```python
from build123d import *

# Parameters (mm, degrees)
BOSS_EXTRUDE1_DEPTH      = 8.83
BOSS_EXTRUDE1_DEPTH_BACK = 3.83
SKETCH1_W                = 35.75
SKETCH1_H                = 30
SKETCH1_R                = 1.725
SKETCH2_W                = 31.75
SKETCH2_H                = 4.83
CUT_EXTRUDE1_DEPTH       = 37.317668183
BOSS_EXTRUDE4_DEPTH      = 7.368601
BOSS_EXTRUDE4_DEPTH_BACK = 22.631399
SKETCH7_W                = 25.4
SKETCH7_H                = 1.05
CUT_EXTRUDE2_DEPTH       = 73.49839785
SKETCH8_R                = 2.85
CUT_EXTRUDE3_DEPTH       = 3


with BuildPart() as part:
    # Sketch1 → Boss-Extrude1 (new, two sides: drawn at the far end of the back side and taken through both)
    with BuildSketch(Plane(origin=(0, 0, 0), x_dir=(1, 0, 0), z_dir=(0, 1, 0)).offset(-BOSS_EXTRUDE1_DEPTH_BACK)):
        with Locations((-0.591296928, 7.631399317)):
            Rectangle(SKETCH1_W, SKETCH1_H)
        with Locations(Location((-0.591296928, 7.631399317, 0), (0, 0, 270))):
            Circle(SKETCH1_R, mode=Mode.SUBTRACT)
    extrude(amount=BOSS_EXTRUDE1_DEPTH + BOSS_EXTRUDE1_DEPTH_BACK)

    # Sketch2 → Cut-Extrude1 (cut, through all)
    with BuildSketch(Plane(origin=(0, 0, -22.631399317), x_dir=(-1, 0, 0), z_dir=(0, 0, -1))):
        with Locations((0.591296928, 2.5)):
            Rectangle(SKETCH2_W, SKETCH2_H)
    extrude(amount=-CUT_EXTRUDE1_DEPTH, mode=Mode.SUBTRACT)

    # Sketch4 → Boss-Extrude4 (add, two sides: drawn at the far end of the back side and taken through both)
    with BuildSketch(Plane.XY.offset(-BOSS_EXTRUDE4_DEPTH_BACK)):
        with BuildLine():
            Line((33.562284713, -6.212446851), (19.98770661, -6.212446851))
            ThreePointArc((19.98770661, -6.212446851), (18.67257107, -4.979381394), (17.283703072, -3.83))
            Line((17.283703072, -3.83), (17.283703072, 8.83))
            ThreePointArc((17.283703072, 8.83), (26.488439568, 2.461776787), (33.562284713, -6.212446851))
        make_face()
        with BuildLine():
            Line((-21.170300466, -6.212446851), (-34.74487857, -6.212446851))
            ThreePointArc((-34.74487857, -6.212446851), (-27.671033425, 2.461776787), (-18.466296928, 8.83))
            Line((-18.466296928, 8.83), (-18.466296928, -3.83))
            ThreePointArc((-18.466296928, -3.83), (-19.855164927, -4.979381394), (-21.170300466, -6.212446851))
        make_face()
    extrude(amount=BOSS_EXTRUDE4_DEPTH + BOSS_EXTRUDE4_DEPTH_BACK)

    # Sketch7 → Cut-Extrude2 (cut, through all)
    with BuildSketch(Plane.ZY.offset(34.74487857)):
        with Locations((-7.631399317, -4.340632565)):
            Rectangle(SKETCH7_W, SKETCH7_H)
    extrude(amount=-CUT_EXTRUDE2_DEPTH, mode=Mode.SUBTRACT)

    # Sketch8 → Cut-Extrude3 (cut)
    with BuildSketch(Plane.XZ.offset(3.83)):
        with Locations(Location((-0.591296928, -7.631399317, 0), (0, 0, 270))):
            Circle(SKETCH8_R)
    extrude(amount=-CUT_EXTRUDE3_DEPTH, mode=Mode.SUBTRACT)


solid = part.part
```
The model under review builds one solid part; all positions refer to its coordinate system, in mm. A direction names the side the tool comes from. Round coordinates to 2 decimals unless told otherwise and drop trailing zeros. Write each loop counter-clockwise with the first axis right and the second up, starting at its lowest first coordinate (ties: lowest second). Pieces come first, ordered by that corner, then holes. Notation, with made-up numbers: (-10.75, -33) - (-5.75, -33) arc R13 cw to (-5.75, -17) - close; hole circle Ø5 at (35, 81). An arc over 180 degrees is marked (long way). Answer as CSV lines item,"result". Start each with the question number.
(1) Draft analysis for pull direction Y (two halves, no side actions). For faces 6 (the flat face through (-16.466, 2, -8)), 7 (the cylindrical face through (-1.252, -0.379, -6.038)), 8 (the flat face through (-1, -3.83, 6)), state which applies: pulls with the +Y half, pulls with the -Y half, needs draft (parallel to the pull), parting line crosses it, or undercut.
(2) For pin 1 Ø2 at (y, z) = (5, -15.5) entering from +X; pin 2 Ø15 at (x, z) = (6, -3) entering from -Y; pin 3 Ø4 at (x, z) = (17, -2) entering from -Y; pin 4 Ø0.5 at (x, y) = (10, -4.5) entering from +Z, all flat-tipped, find the tip position at first contact; note any pin that passes through.
(3) To check wall thickness, follow line 1 (Y direction, x = 8, z = -12) (3 decimals); line 2 (Y direction, x = 17, z = -10.5); line 3 (X direction, y = 8.25, z = -8.5). State the ranges of each line that lie inside material, in increasing order.
(4) For faces 1 (the flat face through (-1, -3.83, -21)), 2 (the flat face through (15.284, 2, -8)), 3 (the flat face through (-2, -0.83, -9)), 4 (the flat face through (-1, -3.816, -11)), 5 (the flat face through (-1, 8.83, -11)), list the 3-axis set-ups (+Z, -Z, +X, -X, +Y, -Y) from which the entire face can be reached by the end or side of a thin tool; tool diameter is ignored.
(5) We need section C-C on y = 3. State the section outline as (x, z) points, plus the area to 3 significant figures.
(6) We need section A-A on z = -14. State the section outline as (x, y) points (3 decimals).
(7) We need section B-B on x = 13.5. State the section outline as (y, z) points (3 decimals).
(8) We need section D-D on z = -8. State the section outline as (x, y) points (3 decimals).
Worked answers:
1,face 6,"undercut"
1,face 7,"needs draft"
1,face 8,"pulls with the -Y half"
2,pin 1,"x = 24.72"
2,pin 2,"y = -3.82"
2,pin 3,"y = -5.27"
2,pin 4,"through"
3,line 1,"-3.816 to 0.085, 4.915 to 8.83"
3,line 2,"-3.82 to 8.83"
3,line 3,"-19.58 to -2.08, 0.9 to 18.4"
4,face 1,"+Z, -Z, -Y"
4,face 2,"+Z, -Z"
4,face 3,"-Y"
4,face 4,"+X, -X"
4,face 5,"+Z, -Z, +X, -X, +Y"
5,outline,"(-27.08, -22.63) - (-16.47, -22.63) - (-16.47, 7.37) - (-27.08, 7.37) - close; (15.28, -22.63) - (25.89, -22.63) - (25.89, 7.37) - (15.28, 7.37) - close"
5,area,"637 mm²"
6,outline,"(-34.745, -6.212) - (-21.17, -6.212) arc R29.14 cw to (-19.725, -4.866) - (-33.894, -4.866) arc R39.901 ccw to start; (-33.177, -3.816) - (31.994, -3.816) arc R39.901 ccw to (17.284, 8.83) - (-18.466, 8.83) arc R39.901 ccw to start; (18.543, -4.866) arc R29.14 cw to (19.988, -6.212) - (33.562, -6.212) arc R39.901 ccw to (32.712, -4.866) - close; hole (-16.466, 0.085) - (15.284, 0.085) - (15.284, 4.915) - (-16.466, 4.915) - close"
7,outline,"(-3.83, -22.631) - (0.085, -22.631) - (0.085, 7.369) - (-3.83, 7.369) - (-3.83, 5.069) - (-3.816, 5.069) - (-3.816, -20.331) - (-3.83, -20.331) - close; (4.915, -22.631) - (8.83, -22.631) - (8.83, 7.369) - (4.915, 7.369) - close"
8,outline,"(-34.745, -6.212) - (-21.17, -6.212) arc R29.14 cw to (-19.725, -4.866) - (-33.894, -4.866) arc R39.901 ccw to start; (-33.177, -3.816) - (-3.417, -3.816) - (-3.417, -0.83) - (-2.276, -0.83) - (-2.276, 0.085) - (-16.466, 0.085) - (-16.466, 4.915) - (-2.276, 4.915) - (-2.276, 8.83) - (-18.466, 8.83) arc R39.901 ccw to start; (1.094, -0.83) - (2.235, -0.83) - (2.235, -3.816) - (31.994, -3.816) arc R39.901 ccw to (17.284, 8.83) - (1.094, 8.83) - (1.094, 4.915) - (15.284, 4.915) - (15.284, 0.085) - (1.094, 0.085) - close; (18.543, -4.866) arc R29.14 cw to (19.988, -6.212) - (33.562, -6.212) arc R39.901 ccw to (32.712, -4.866) - close"
